from build123d import *

# Parameters (mm, degrees)
F0_R     = 15.875
F1_DEPTH = 6.35
F2_R     = 9.525
F3_DEPTH = 62.23
F4_SIZE  = 1.27
F5_R     = 2.3876
F6_DEPTH = 15.876
F7_R     = 2.3876
F8_DEPTH = 15.876


with BuildPart() as f1:
    # F0 (on Right) → F1 (new body)
    with BuildSketch(Plane.YZ):
        Circle(F0_R)
    extrude(amount=F1_DEPTH)

    # F2 (on face) → F3 (join)
    with BuildSketch(Plane.YZ.offset(6.35)):
        Circle(F2_R)
    extrude(amount=F3_DEPTH)

    # F4
    f4_edges = [f1.edges().sort_by_distance(p)[0] for p in [
        (68.58, -9.525, 0),
    ]]
    chamfer(f4_edges, length=F4_SIZE)

    # F5 (on Front) → F6 (cut, through all)
    with BuildSketch(Plane.XZ):
        with Locations((62.23, 0)):
            Circle(F5_R)
    extrude(amount=-F6_DEPTH, mode=Mode.SUBTRACT)

    # F7 (on face) → F8 (cut, through all)
    with BuildSketch(Plane(origin=(0, 0, 0), x_dir=(-1, 0, 0), z_dir=(0, 1, 0))):
        with Locations((-62.23, 0)):
            Circle(F7_R)
    extrude(amount=-F8_DEPTH, mode=Mode.SUBTRACT)


solid = f1.part
Check sheet for the modelled part. Datum: model origin and axes. Units: mm. A direction names the side the tool comes from. Coordinates: 2 decimals unless noted, no trailing zeros. Write each loop counter-clockwise with the first axis right and the second up, starting at its lowest first coordinate (ties: lowest second). Pieces come first, ordered by that corner, then holes. Notation, with made-up numbers: M 3,54 L 34,54 A10 cw 34,71 Z; hole C -35,24.25 d11. An arc over 180 degrees is marked long. Answer as CSV lines item,"result".
Q1. Set-up check for faces 1 (the face through (3.131, -3.441, -15.497)), 2 (the face through (6.35, 7, -7)): record each of +Z, -Z, +X, -X, +Y, -Y from which the full face is reachable in a straight line by a thin tool's end or side.
Check result:
face 1,"+X, -X"
face 2,"+X"
Q2. Cross-section at B-B (x = 62.23). Record the boundary of the cut face in (y, z) (3 decimals), then the cut area to 3 significant figures.
Check result:
outline,"M -9.221,-2.388 A9.525 ccw 9.221,-2.388 Z; M -9.221,2.388 L 9.221,2.388 A9.525 ccw Z"
area,"195 mm^2"
Q3. Cross-section at A-A (z = 0). Record the boundary of the cut face in (x, y) (3 decimals), then the cut area to 3 significant figures.
Check result:
outline,"M 0,-15.875 L 6.35,-15.875 L 6.35,-9.525 L 59.842,-9.525 L 59.842,9.525 L 6.35,9.525 L 6.35,15.875 L 0,15.875 Z; M 64.618,-9.525 L 67.31,-9.525 L 68.58,-8.255 L 68.58,8.255 L 67.31,9.525 L 64.618,9.525 Z"
area,"1,290 mm^2"
Q4. Go/stop test with flat-tipped pins: pin 1 (10 mm diameter, centred on x = 29.5, y = -10.5, fed in from +Z); pin 2 (6 mm diameter, centred on x = 30, y = -8, fed in from +Z); pin 3 (1 mm diameter, centred on x = 37.5, z = 4, fed in from -Y); pin 4 (3 mm diameter, centred on x = 62.23, z = 0, fed in from -Y). Record where each tip stops, or that it passes through.
Check result:
pin 1,"z = 7.78"
pin 2,"z = 8.11"
pin 3,"y = -8.86"
pin 4,"through"
Q5. Material ranges on probe 1 along X at (y, z) = (3.25, 0); probe 2 along X at (y, z) = (11.5, -10); probe 3 along Z at (x, y) = (62.23, 7), recorded low to high. Write a range as from..to.
Check result:
probe 1,"0..59.84, 64.62..68.58"
probe 2,"0..6.35"
probe 3,"-6.46..-2.39, 2.39..6.46"
Q6. Cross-section at D-D (z = -12.5). Record the boundary of the cut face in (x, y), then the cut area to 3 significant figures.
Check result:
outline,"M 0,-9.79 L 6.35,-9.79 L 6.35,9.79 L 0,9.79 Z"
area,"124 mm^2"
Q7. Cross-section at C-C (x = 13.5). Record the boundary of the cut face in (y, z) (3 decimals), then the cut area to 3 significant figures.
Check result:
outline,"C 0,0 d19.05"
area,"285 mm^2"
